Geometry check sheet. Reference: the model listing, model coordinates, mm. A direction names the side the tool comes from. Coordinates: 2 decimals unless noted, no trailing zeros. Loops run counter-clockwise (first coordinate to the right, second up) from the corner with the lowest first, then second, coordinate; pieces in that order, holes last.
Autodesk Inventor part; units mm, degrees
ref_plane "YZ Plane" through (0, 0, 0) normal (1, 0, 0) x (0, 1, 0)
ref_plane "XZ Plane" through (0, 0, 0) normal (0, 1, 0) x (-1, 0, 0)
ref_plane "XY Plane" through (0, 0, 0) normal (0, 0, 1) x (1, 0, 0)
sketch "Náčrt1" plane through (0, 0, 0) normal (0, 0, 1) x (1, 0, 0)
  circle A0 centre (0, 0) radius 12.5
  dimension "d0" = 25
extrude "Vysunutí1" add sketch "Náčrt1" along normal blind 30
sketch "Náčrt2" plane through (0, 0, 30) normal (0, 0, 1) x (1, 0, 0)
  circle A0 centre (0, 0) radius 15
  dimension "d3" = 30
extrude "Vysunutí2" add sketch "Náčrt2" along normal blind 80
sketch "Náčrt3" plane through (0, 0, 110) normal (0, 0, 1) x (1, 0, 0)
  circle A0 centre (0, 0) radius 12.5
  dimension "d6" = 25
extrude "Vysunutí3" add sketch "Náčrt3" along normal blind 70
sketch "Náčrt4" plane through (0, 0, 0) normal (1, 0, 0) x (0, 1, 0)
  point P0 (0, 0)
sketch "Náčrt5" plane through (0, 0, 0) normal (0, 1, 0) x (-1, 0, 0)
  line L0 (0, -36) -> (0, 216) construction
  arc A0 (-4, 38.6) -> (4, 38.6) centre (0, 38.6) ccw
  line L1 (-15, 30) -> (15, 30) construction
  arc A1 (4, 70.6) -> (-4, 70.6) centre (0, 70.6) ccw
  line L2 (4, 70.6) -> (4, 38.6)
  line L3 (-4, 70.6) -> (-4, 38.6)
  point P0 (0, 0)
  dimension "d9" = 8
  dimension "d10" = 8.6
  dimension "d11" = 8
  dimension "d12" = 32
properties part number "Součást3"
1) Depth check by flat-ended pin: pin 1 (5 mm diameter, centred on y = 6, z = 38.5, fed in from -X); pin 2 (4 mm diameter, centred on y = -6, z = 72, fed in from +X); pin 3 (1.5 mm diameter, centred on y = 1.5, z = 89, fed in from -X). Enter the tip coordinate at first touch or a pass-through.
Data:
pin 1: stops at x = -14.59
pin 2: stops at x = 14.46
pin 3: stops at x = -14.98
2) Access from +Z, -Z, +X, -X, +Y, -Y to the whole of each face (thin tool, end or side, straight path). Record for faces 1 (the flat face through (-3.4, 12.3, 110)), 2 (the flat face through (0, 0, 0)), 3 (the cylindrical face through (11.923, -3.755, 14.79)).
Data:
face 1: +Z
face 2: -Z, +X, -X, +Y, -Y
face 3: -Z
3) Material ranges on probe 1 along Y at (x, z) = (-0.5, 155); probe 2 along Z at (x, y) = (12.5, 8); probe 3 along Y at (x, z) = (2.75, 103.5), recorded low to high.
Data:
probe 1: y = -12.49 to 12.49
probe 2: z = 30 to 110
probe 3: y = -14.75 to 14.75
4) Section check C-C on z = 24. Record the cut outline in (x, y), and give its area (3 significant figures).
Data:
outline: circle Ø25 at (0, 0)
area: 491 mm2
5) Section check D-D on z = 82. Record the cut outline in (x, y), and give its area (3 significant figures).
Data:
outline: circle Ø30 at (0, 0)
area: 707 mm2
6) Section check A-A on y = 0. Record the cut outline in (x, z), and give its area (3 significant figures).
Data:
outline: (-15, 30) - (-12.5, 30) - (-12.5, 0) - (12.5, 0) - (12.5, 30) - (15, 30) - (15, 110) - (12.5, 110) - (12.5, 180) - (-12.5, 180) - (-12.5, 110) - (-15, 110) - close
area: 4,900 mm2
